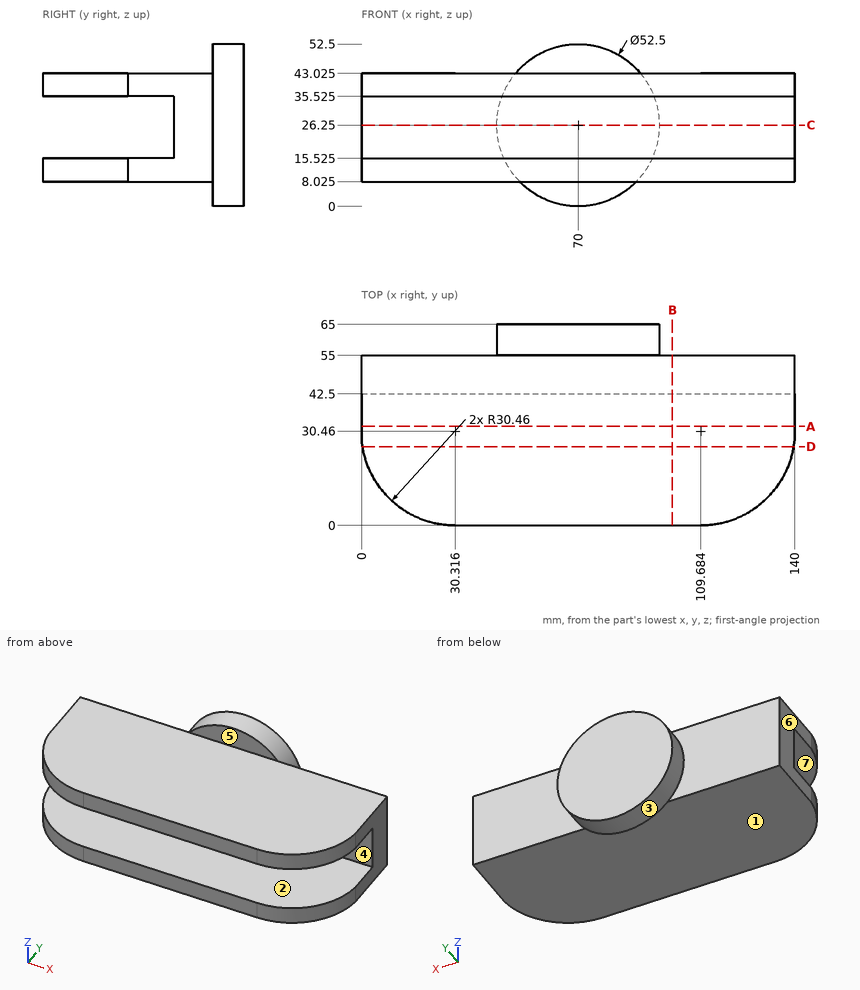
Source: three-view drawing plus pictorial views. Frame: mm from the lowest corner of the part. A direction names the side the tool comes from. Coordinates: 2 decimals unless noted, no trailing zeros. Loops run counter-clockwise (first coordinate to the right, second up) from the corner with the lowest first, then second, coordinate; pieces in that order, holes last. Notation, with made-up numbers: (-28, -34) -> (1, -34) arc R15 cw to (1, -21) -> close; hole circle Ø4 at (31.5, -12.5). An arc over 180 degrees is marked (long way). Write each question's results on one line, items separated by ' | '. Start each with the question number.
Q1. Reachability of the marked faces 5, 6 and 7 from +Z, -Z, +X, -X, +Y, -Y: full face, straight path, thin tool, end or side. Return the list, or none.
Q2. Pin query (flat end, axial travel): pin 1 (10 mm diameter, centred on y = 10, z = 41, fed in from +X); pin 2 (10.5 mm diameter, centred on x = 72, z = 50, fed in from -Y); pin 3 (10.5 mm diameter, centred on x = 108.5, z = 21, fed in from +Y). Return the tip coordinate at first contact, or that it passes through.
Q3. Pull-direction query (Z, two-part tool) for the marked faces 1, 2, 3 and 4; classes: released by +Z, released by -Z, zero draft, split by the parting line, or undercut.
Q4. Section D-D, the plane y = 25.5. Return the cut outline in (x, z) (1 decimal).
Q5. Ray query, line 1 (Z direction, x = 73.5, y = 39) (1 decimal); line 2 (Z direction, x = 53, y = 51.5) (1 decimal); line 3 (Y direction, x = 96.5, z = 21). Return the intervals inside material, ascending. Write a range as from..to.
Q6. Section B-B, the plane x = 100.5. Return the cut outline in (y, z) (1 decimal), plus the area to 4 significant figures.
Q7. Section A-A, the plane y = 32. Return the cut outline in (x, z) (1 decimal), plus the area to 3 significant figures.
Q8. Section C-C, the plane z = 26.25. Return the cut outline in (x, y).
Found:
1) face 5: +Z, +X, -X, -Y | face 6: +Z, -Z, -X, +Y, -Y | face 7: +X, -X, -Y
2) pin 1: x = 135.93 | pin 2: y = 55 | pin 3: y = 55
3) face 1: released by -Z | face 2: undercut | face 3: split by the parting line | face 4: undercut
4) outline: (0.3, 8) -> (139.7, 8) -> (139.7, 15.5) -> (0.3, 15.5) -> close; (0.3, 35.5) -> (139.7, 35.5) -> (139.7, 43) -> (0.3, 43) -> close
5) line 1: 8..15.5, 35.5..43 | line 2: 8..43 | line 3: 42.5..55
6) outline: (0, 8) -> (55, 8) -> (55, 43) -> (0, 43) -> (0, 35.5) -> (42.5, 35.5) -> (42.5, 15.5) -> (0, 15.5) -> close | area: 1,075 mm2
7) outline: (0, 8) -> (140, 8) -> (140, 15.5) -> (0, 15.5) -> close; (0, 35.5) -> (140, 35.5) -> (140, 43) -> (0, 43) -> close | area: 2,100 mm2
8) outline: (0, 42.5) -> (140, 42.5) -> (140, 55) -> (96.25, 55) -> (96.25, 65) -> (43.75, 65) -> (43.75, 55) -> (0, 55) -> close
